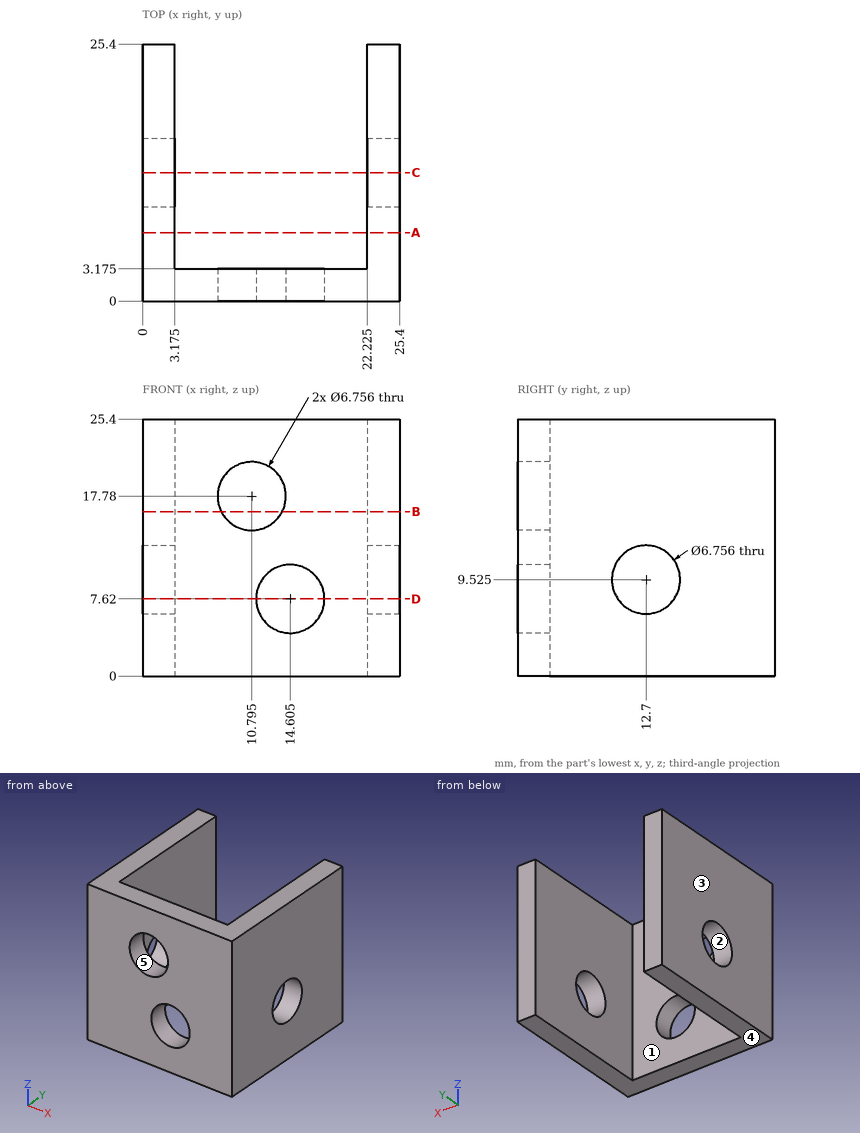
Can you work these out from the drawing? Everything is in mm from the part's minimum corner. A direction names the side the tool comes from. Round coordinates to 2 decimals unless told otherwise and drop trailing zeros. Loops run counter-clockwise (first coordinate to the right, second up) from the corner with the lowest first, then second, coordinate; pieces in that order, holes last. Notation, with made-up numbers: (61.5, -14) -> (114.5, -14) arc R16 cw to (114.5, -5) -> close; hole circle Ø4 at (-33, 50). An arc over 180 degrees is marked (long way). One line per question, with ' | ' between items.
(1) If I drill on probe 1 along X at (y, z) = (4.25, 4.5) (1 decimal); probe 2 along X at (y, z) = (1.35, 17.78); probe 3 along Y at (x, z) = (9.75, 8.25) (1 decimal), over which ranges is the centre line in solid material (lowest first)?
Model answer:
probe 1: x = 0 to 3.2, 22.2 to 25.4 | probe 2: x = 0 to 7.42, 14.17 to 25.4 | probe 3: y = 0 to 3.2
(2) Thinking about a two-plate mould opening in X: for the marked faces 3, 4 and 5, which applies, released by +X, released by -X, zero draft, split by the parting line, or undercut?
Model answer:
face 3: released by -X | face 4: zero draft | face 5: undercut
(3) If we section it at A-A on y = 6.75: List the corners of the cut face in (x, z) for me (1 decimal).
Model answer:
outline: (0, 0) -> (3.2, 0) -> (3.2, 25.4) -> (0, 25.4) -> close; (22.2, 0) -> (25.4, 0) -> (25.4, 25.4) -> (22.2, 25.4) -> close
(4) For the marked faces 1 and 2, which set-ups out of +Z, -Z, +X, -X, +Y, -Y let a thin tool reach every point of the face, with its end or its side?
Model answer:
face 1: +Z, -Z, +Y | face 2: +X, -X
(5) If we section it at D-D on z = 7.62: List the corners of the cut face in (x, y) for me (1 decimal).
Model answer:
outline: (0, 0) -> (11.2, 0) -> (11.2, 3.2) -> (3.2, 3.2) -> (3.2, 9.9) -> (0, 9.9) -> close; (0, 15.5) -> (3.2, 15.5) -> (3.2, 25.4) -> (0, 25.4) -> close; (18, 0) -> (25.4, 0) -> (25.4, 9.9) -> (22.2, 9.9) -> (22.2, 3.2) -> (18, 3.2) -> close; (22.2, 15.5) -> (25.4, 15.5) -> (25.4, 25.4) -> (22.2, 25.4) -> close
(6) If we section it at B-B on z = 16.25: List the corners of the cut face in (x, y) for me (1 decimal), and give its area (3 significant figures).
Model answer:
outline: (0, 0) -> (7.8, 0) -> (7.8, 3.2) -> (3.2, 3.2) -> (3.2, 25.4) -> (0, 25.4) -> close; (13.8, 0) -> (25.4, 0) -> (25.4, 25.4) -> (22.2, 25.4) -> (22.2, 3.2) -> (13.8, 3.2) -> close | area: 203 mm^2
(7) If we section it at C-C on y = 12.7: List the corners of the cut face in (x, z) for me (1 decimal).
Model answer:
outline: (0, 0) -> (3.2, 0) -> (3.2, 6.1) -> (0, 6.1) -> close; (0, 12.9) -> (3.2, 12.9) -> (3.2, 25.4) -> (0, 25.4) -> close; (22.2, 0) -> (25.4, 0) -> (25.4, 6.1) -> (22.2, 6.1) -> close; (22.2, 12.9) -> (25.4, 12.9) -> (25.4, 25.4) -> (22.2, 25.4) -> close
(8) For pin 1 Ø6 at (x, y) = (9, 17.5) entering from +Z; pin 2 Ø5.5 at (x, z) = (14, 16.5) entering from +Y (3 decimals), each with a flat end and sliding along its axis, tell me the tip position at first contact or that it passes through.
Model answer:
pin 1: passes through | pin 2: stops at y = 3.175
